```python
from build123d import *

# Parameters (mm, degrees)
SKETCH1_R           = 20
SKETCH1_R_2         = 11
BOSS_EXTRUDE1_DEPTH = 44
BOSS_EXTRUDE2_DEPTH = 44
CUT_EXTRUDE1_DEPTH  = 44
BOSS_EXTRUDE3_DEPTH = 2
SKETCH4_R           = 6
CUT_EXTRUDE2_DEPTH  = 44


with BuildPart() as part:
    # Sketch1 → Boss-Extrude1 (new body)
    with BuildSketch(Plane.XY):
        with Locations((-57.809139785, 0)):
            Circle(SKETCH1_R)
        with Locations((-57.809139785, 0)):
            Circle(SKETCH1_R_2, mode=Mode.SUBTRACT)
    extrude(amount=BOSS_EXTRUDE1_DEPTH)

    # Sketch1_5 → Boss-Extrude2 (add)
    with BuildSketch(Plane.XY):
        with BuildLine():
            ThreePointArc((-38.444223054, -5), (-45.561691071, -15.811388301), (-57.809139785, -20))
            Line((-57.809139785, -20), (47.190860215, -20))
            Line((47.190860215, -20), (47.190860215, -5))
            Line((47.190860215, -5), (-38.444223054, -5))
        make_face()
    extrude(amount=BOSS_EXTRUDE2_DEPTH)

    # Sketch2 → Cut-Extrude1 (cut)
    with BuildSketch(Plane(origin=(0, -5, 0), x_dir=(1, 0, 0), z_dir=(0, 1, 0))):
        with BuildLine():
            Line((47.190860215, -42), (47.190860215, -22))
            ThreePointArc((47.190860215, -22), (41.332995839, -36.142135624), (27.190860215, -42))
            Line((27.190860215, -42), (47.190860215, -42))
        make_face()
        with BuildLine():
            Line((47.190860215, -2), (27.190860215, -2))
            ThreePointArc((27.190860215, -2), (41.332995839, -7.857864376), (47.190860215, -22))
            Line((47.190860215, -22), (47.190860215, -2))
        make_face()
        Polygon((27.190860215, -42), (-38.444223054, -42), (-38.444223054, -44), (47.190860215, -44), (47.190860215, -42), align=None)
        Polygon((47.190860215, 0), (-38.444223054, 0), (-38.444223054, -2), (27.190860215, -2), (47.190860215, -2), align=None)
    extrude(amount=-CUT_EXTRUDE1_DEPTH, mode=Mode.SUBTRACT)

    # Sketch3 → Boss-Extrude3 (add)
    with BuildSketch(Plane(origin=(0, -5, 0), x_dir=(1, 0, 0), z_dir=(0, 1, 0))):
        with BuildLine():
            Line((27.190860215, -7), (-7.809139785, -7))
            ThreePointArc((-7.809139785, -7), (-22.809139785, -22), (-7.809139785, -37))
            Line((-7.809139785, -37), (27.190860215, -37))
            ThreePointArc((27.190860215, -37), (42.190860215, -22), (27.190860215, -7))
        make_face()
    extrude(amount=BOSS_EXTRUDE3_DEPTH)

    # Sketch4 → Cut-Extrude2 (cut)
    with BuildSketch(Plane(origin=(0, -3, 0), x_dir=(1, 0, 0), z_dir=(0, 1, 0))):
        with Locations((27.190860215, -22)):
            Circle(SKETCH4_R)
        with Locations((-7.809139785, -22)):
            Circle(SKETCH4_R)
    extrude(amount=-CUT_EXTRUDE2_DEPTH, mode=Mode.SUBTRACT)


solid = part.part
```
The model under review builds one solid part; all positions refer to its coordinate system, in mm. A direction names the side the tool comes from. Round coordinates to 2 decimals unless told otherwise and drop trailing zeros. Write each loop counter-clockwise with the first axis right and the second up, starting at its lowest first coordinate (ties: lowest second). Pieces come first, ordered by that corner, then holes. Notation, with made-up numbers: (-36, 18.5) - (15, 18.5) arc R34 ccw to (15, 55.5) - close; hole circle Ø9 at (-16, 46). An arc over 180 degrees is marked (long way). Answer as CSV lines item,"result". Start each with the question number.
(1) To check wall thickness, follow line 1 (Y direction, x = 34.5, z = 8); line 2 (X direction, y = -15.5, z = 22); line 3 (X direction, y = -10, z = 25.5). State the ranges of each line that lie inside material, in increasing order.
(2) We need section D-D on y = -9.5. State the section outline as (x, z) points, plus the area to 3 significant figures.
(3) We need section B-B on x = 16. State the section outline as (y, z) points.
(4) For faces 1 (the flat face through (9, -3, 22)), 2 (the cylindrical face through (-22.806, -4.014, 21.67)), 3 (the cylindrical face through (42.187, -4.014, 22.33)), list the 3-axis set-ups (+Z, -Z, +X, -X, +Y, -Y) from which the entire face can be reached by the end or side of a thin tool; tool diameter is ignored.
(5) We need section A-A on y = 0. State the section outline as (x, z) points, plus the area to 3 significant figures.
(6) Draft analysis for pull direction Z (two halves, no side actions). For faces 4 (the flat face through (-6, -12, 2)), 5 (the flat face through (-5, -12, 42)), 6 (the cylindrical face through (-13.8, -11.4, 21.7)), 7 (the cylindrical face through (32.914, -11.381, 20.198)), state which applies: pulls with the +Z half, pulls with the -Z half, needs draft (parallel to the pull), parting line crosses it, or undercut.
(7) We need section C-C on z = 33. State the section outline as (x, y) points, plus the area to 3 significant figures.
(8) For pin 1 Ø3 at (y, z) = (13.5, 23.5) entering from +X; pin 2 Ø2 at (y, z) = (-15.5, 43.5) entering from +X; pin 3 Ø19 at (x, z) = (-7.81, 22) entering from +Y; pin 4 Ø17.5 at (x, y) = (-57.81, 0) entering from +Z, all flat-tipped, find the tip position at first contact; note any pin that passes through.
Worked answers:
1,line 1,"-20 to -5"
1,line 2,"-70.45 to -13.81, -1.81 to 21.19, 33.19 to 47.19"
1,line 3,"-75.13 to -62.39, -53.23 to -12.68, -2.94 to 22.32, 32.06 to 46.88"
2,outline,"(-75.41, 0) - (-63.35, 0) - (-63.35, 44) - (-75.41, 44) - close; (-52.26, 0) - (-38.44, 0) - (-38.44, 2) - (27.19, 2) arc R20 ccw to (27.19, 42) - (-38.44, 42) - (-38.44, 44) - (-52.26, 44) - close; hole circle Ø12 at (-7.81, 22); hole circle Ø12 at (27.19, 22)"
2,area,"4,170 mm²"
3,outline,"(-20, 2) - (-5, 2) - (-5, 7) - (-3, 7) - (-3, 37) - (-5, 37) - (-5, 42) - (-20, 42) - close"
4,face 1,"+Z, -Z, +X, +Y"
4,face 2,"+Y"
4,face 3,"+X, +Y"
5,outline,"(-77.81, 0) - (-68.81, 0) - (-68.81, 44) - (-77.81, 44) - close; (-46.81, 0) - (-37.81, 0) - (-37.81, 44) - (-46.81, 44) - close"
5,area,"792 mm²"
6,face 4,"pulls with the -Z half"
6,face 5,"pulls with the +Z half"
6,face 6,"undercut"
6,face 7,"undercut"
7,outline,"(-57.81, -20) - (43.89, -20) - (43.89, -5) - (37.39, -5) - (37.39, -3) - (-18.01, -3) - (-18.01, -5) - (-38.44, -5) arc R20 ccw (long way) to start; hole circle Ø22 at (-57.81, 0)"
7,area,"2,300 mm²"
8,pin 1,"x = -41.81"
8,pin 2,"x = -38.44"
8,pin 3,"y = -3"
8,pin 4,"through"
